Geometry check sheet. Reference: the model listing, model coordinates, mm. Face numbers are marked on the shaded views. A direction names the side the tool comes from. Give positions to 0.01 mm unless a question says otherwise; leave off trailing zeros. Loops run counter-clockwise (first coordinate to the right, second up) from the corner with the lowest first, then second, coordinate; pieces in that order, holes last. Notation, with made-up numbers: (51.25, -1.75) -> (58.25, -1.75) arc R4 ccw to (58.25, 2.25) -> close; hole circle Ø9 at (-37.5, 70). An arc over 180 degrees is marked (long way). Answer in a Markdown table with one row per item. Add a question column.
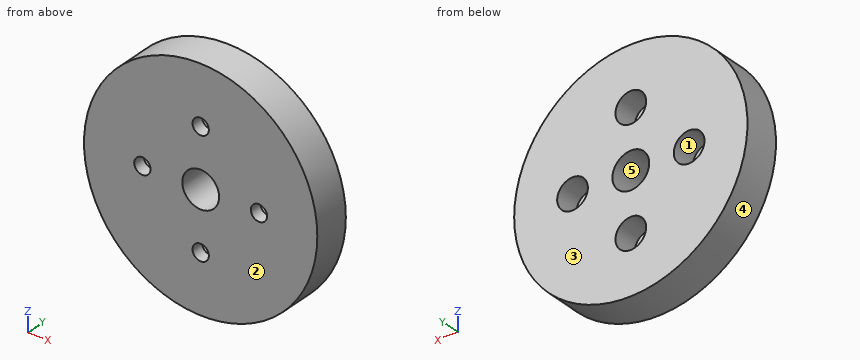
```python
from build123d import *

# Parameters (mm, degrees)
F0_R           = 60.325
F1_DEPTH       = 19.05
F3_D           = 8.4328
F3_CBORE_D     = 15.875
F3_CBORE_DEPTH = 12.7
F4_R           = 9.525
F5_DEPTH       = 25.4


with BuildPart() as f1:
    # F0 (on Front) → F1 (new body)
    with BuildSketch(Plane.XZ):
        Circle(F0_R)
    extrude(amount=-F1_DEPTH)

    # F3 (through all)
    with Locations(Plane(origin=(0, 19.05, 0), x_dir=(-1, 0, 0), z_dir=(0, 1, 0))):
        with Locations((0, 30.1498), (30.1498, 0), (0, -30.1498), (-30.1498, 0)):
            CounterBoreHole(F3_D / 2, F3_CBORE_D / 2, F3_CBORE_DEPTH)

    # F4 (on face) → F5 (cut)
    with BuildSketch(Plane(origin=(0, 19.05, 0), x_dir=(-1, 0, 0), z_dir=(0, 1, 0))):
        Circle(F4_R)
    extrude(amount=-F5_DEPTH, mode=Mode.SUBTRACT)


solid = f1.part
```
1. Release check for a two-part mould opening along Z. For the marked faces 3, 4 and 5 record: released by +Z, released by -Z, zero draft, split by the parting line, or undercut.
2. Sectioned sample at D-D (z = 51.5). Enter the section's corners in (x, y).
3. Sectioned sample at B-B (z = 0). Enter the section's corners in (x, y) (3 decimals), plus the area to 3 significant figures.
4. Sectioned sample at A-A (x = 0). Enter the section's corners in (y, z) (3 decimals).
5. Material ranges on L1, parallel to Z at x = 0, y = 15.75 (3 decimals); L2, parallel to Z at x = 0, y = 2.5 (3 decimals); L3, parallel to X at y = 16, z = 6, recorded low to high. Write a range as from..to.
6. Sectioned sample at C-C (y = 17). Count the separate pieces of the cut face and the enclosed holes in it, plus the area to 3 significant figures.
7. Gauge pin test, flat ends, axial feed: pin 1 Ø12 at (x, z) = (-24.5, -45) entering from -Y; pin 2 Ø5 at (x, z) = (32, 3) entering from +Y; pin 3 Ø3 at (y, z) = (10, 7.5) entering from -X; pin 4 Ø5 at (y, z) = (5.5, -17.5) entering from -X. Record the tip position at first contact, or that the pin passes through.
8. Access from +Z, -Z, +X, -X, +Y, -Y to the whole of each face (thin tool, end or side, straight path). Record for the marked faces 1 and 2.
Response:
| question | item | result |
|---|---|---|
| 1 | face 3 | zero draft |
| 1 | face 4 | split by the parting line |
| 1 | face 5 | undercut |
| 2 | outline | (-31.41, 0) -> (31.41, 0) -> (31.41, 19.05) -> (-31.41, 19.05) -> close |
| 3 | outline | (-60.325, 0) -> (-34.366, 0) -> (-34.366, 6.35) -> (-38.087, 6.35) -> (-38.087, 19.05) -> (-60.325, 19.05) -> close; (-25.933, 0) -> (-9.525, 0) -> (-9.525, 19.05) -> (-22.212, 19.05) -> (-22.212, 6.35) -> (-25.933, 6.35) -> close; (9.525, 0) -> (25.933, 0) -> (25.933, 6.35) -> (22.212, 6.35) -> (22.212, 19.05) -> (9.525, 19.05) -> close; (34.366, 0) -> (60.325, 0) -> (60.325, 19.05) -> (38.087, 19.05) -> (38.087, 6.35) -> (34.366, 6.35) -> close |
| 3 | area | 1,430 mm2 |
| 4 | outline | (0, -60.325) -> (19.05, -60.325) -> (19.05, -38.087) -> (6.35, -38.087) -> (6.35, -34.366) -> (0, -34.366) -> close; (0, -25.933) -> (6.35, -25.933) -> (6.35, -22.212) -> (19.05, -22.212) -> (19.05, -9.525) -> (0, -9.525) -> close; (0, 9.525) -> (19.05, 9.525) -> (19.05, 22.212) -> (6.35, 22.212) -> (6.35, 25.933) -> (0, 25.933) -> close; (0, 34.366) -> (6.35, 34.366) -> (6.35, 38.087) -> (19.05, 38.087) -> (19.05, 60.325) -> (0, 60.325) -> close |
| 5 | L1 | z = -60.325..-38.087, -22.212..-9.525, 9.525..22.212, 38.087..60.325 |
| 5 | L2 | z = -60.325..-34.366, -25.933..-9.525, 9.525..25.933, 34.366..60.325 |
| 5 | L3 | x = -60.03..-35.35, -24.95..-7.4, 7.4..24.95, 35.35..60.03 |
| 6 | separate pieces | 1 |
| 6 | enclosed holes | 5 |
| 6 | area | 10,400 mm2 |
| 7 | pin 1 | stops at y = 0 |
| 7 | pin 2 | stops at y = 6.35 |
| 7 | pin 3 | stops at x = -60.03 |
| 7 | pin 4 | stops at x = -58.43 |
| 8 | face 1 | +Y |
| 8 | face 2 | +Z, -Z, +X, -X, -Y |
